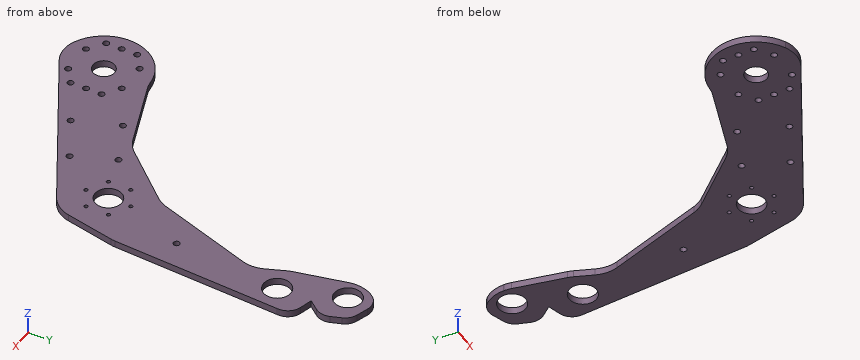
```python
from build123d import *

# Parameters (mm, degrees)
SKETCH1_R           = 8.89
SKETCH1_R_2         = 10.9347
SKETCH1_R_3         = 11.1125
SKETCH1_R_4         = 1.524
SKETCH1_R_5         = 2.5
SKETCH1_R_6         = 2.54
BOSS_EXTRUDE1_DEPTH = 5.55625
FILLET1_R           = 25.4
FILLET3_R           = 12.7
FILLET4_R           = 12.7


with BuildPart() as part:
    # Sketch1 → Boss-Extrude1 (new body)
    with BuildSketch(Plane.XY):
        with BuildLine():
            Line((199.79602437, 71.078107547), (188.964925061, 57.285610842))
            Line((188.964925061, 57.285610842), (206.456809173, 52.506453094))
            Line((206.456809173, 52.506453094), (208.830818929, 45.887219752))
            Line((208.830818929, 45.887219752), (200.684125291, -98.616772294))
            Line((200.684125291, -98.616772294), (189.611167808, -151.385643895))
            Line((189.611167808, -151.385643895), (38.107034572, -236.120024372))
            ThreePointArc((38.107034572, -236.120024372), (1.581834572, -199.594824372), (38.107034572, -163.069624372))
            Line((38.107034572, -163.069624372), (103.261818833, -139.701647224))
            Line((103.261818833, -139.701647224), (147.550432491, -89.7457244))
            Line((147.550432491, -89.7457244), (171.836242771, -16.814689905))
            Line((171.836242771, -16.814689905), (178.189444477, 2.26417003))
            Line((178.189444477, 2.26417003), (167.830043749, 27.447208055))
            Line((167.830043749, 27.447208055), (157.470643022, 73.010133983))
            Line((157.470643022, 73.010133983), (157.470643022, 93.390021886))
            Line((157.470643022, 93.390021886), (170.600142232, 98.791028052))
            Line((170.600142232, 98.791028052), (192.468434241, 91.508954042))
            Line((192.468434241, 91.508954042), (199.79602437, 71.078107547))
        make_face()
        with Locations((38.107034572, -199.594824372)):
            Circle(SKETCH1_R, mode=Mode.SUBTRACT)
        with Locations((161.671727665, -124.770570211)):
            Circle(SKETCH1_R_2, mode=Mode.SUBTRACT)
        with Locations((188.964925061, 29.396113336)):
            Circle(SKETCH1_R_3, mode=Mode.SUBTRACT)
        with Locations((173.035965272, 78.237579188)):
            Circle(SKETCH1_R_3, mode=Mode.SUBTRACT)
        with Locations((161.671727665, -106.355570211)):
            Circle(SKETCH1_R_4, mode=Mode.SUBTRACT)
        with Locations((12.721199582, -186.891028869)):
            Circle(SKETCH1_R_5, mode=Mode.SUBTRACT)
        with Locations((177.619585475, -115.563070211)):
            Circle(SKETCH1_R_4, mode=Mode.SUBTRACT)
        with Locations((177.619585475, -133.978070211)):
            Circle(SKETCH1_R_4, mode=Mode.SUBTRACT)
        with Locations((161.671727665, -143.185570211)):
            Circle(SKETCH1_R_4, mode=Mode.SUBTRACT)
        with Locations((145.723869854, -133.978070211)):
            Circle(SKETCH1_R_4, mode=Mode.SUBTRACT)
        with Locations((145.723869854, -115.563070211)):
            Circle(SKETCH1_R_4, mode=Mode.SUBTRACT)
        with Locations((12.721199582, -199.591028869)):
            Circle(SKETCH1_R_5, mode=Mode.SUBTRACT)
        with Locations((12.721199582, -212.291028869)):
            Circle(SKETCH1_R_5, mode=Mode.SUBTRACT)
        with Locations((25.421199582, -221.588074125)):
            Circle(SKETCH1_R_5, mode=Mode.SUBTRACT)
        with Locations((25.421199582, -177.593983613)):
            Circle(SKETCH1_R_5, mode=Mode.SUBTRACT)
        with Locations((50.821199582, -177.593983613)):
            Circle(SKETCH1_R_5, mode=Mode.SUBTRACT)
        with Locations((63.521199582, -186.891028869)):
            Circle(SKETCH1_R_5, mode=Mode.SUBTRACT)
        with Locations((63.521199582, -199.591028869)):
            Circle(SKETCH1_R_5, mode=Mode.SUBTRACT)
        with Locations((63.521199582, -212.291028869)):
            Circle(SKETCH1_R_5, mode=Mode.SUBTRACT)
        with Locations((50.821199582, -221.588074125)):
            Circle(SKETCH1_R_5, mode=Mode.SUBTRACT)
        with Locations((181.29246285, -57.510690342)):
            Circle(SKETCH1_R_6, mode=Mode.SUBTRACT)
        with Locations((99.96903305, -191.23088449)):
            Circle(SKETCH1_R_6, mode=Mode.SUBTRACT)
        with Locations((134.782371312, -172.083548446)):
            Circle(SKETCH1_R_6, mode=Mode.SUBTRACT)
        with Locations((121.031102699, -139.896498857)):
            Circle(SKETCH1_R_6, mode=Mode.SUBTRACT)
        with Locations((86.391831128, -156.243479537)):
            Circle(SKETCH1_R_6, mode=Mode.SUBTRACT)
    extrude(amount=BOSS_EXTRUDE1_DEPTH)

    # Fillet1
    # the kernel refuses this fillet: 25.4 mm, written as the material it adds along each edge
    with BuildSketch(Plane(origin=(178.189444477, 2.26417003, 0), x_dir=(-0.38043310119112633, 0.9248084426074961, 0), z_dir=(0, 0, 1))) as fillet1_piece_1:
        with BuildLine():
            CenterArc((FILLET1_R * 0.371679258358, FILLET1_R), FILLET1_R, 229.221887669, 40.778112331)
            Line((-FILLET1_R * 0.281452116845, FILLET1_R * 0.242755385146), (0, 0))
            Line((0, 0), (FILLET1_R * 0.371679258358, 0))
        make_face()
    extrude(amount=5.55625)
    with BuildSketch(Plane(origin=(147.550432491, -89.7457244, 0), x_dir=(0.3159404927300864, 0.9487790074898739, 0), z_dir=(0, 0, 1))) as fillet1_piece_2:
        with BuildLine():
            CenterArc((FILLET1_R * 0.204735054156, FILLET1_R), FILLET1_R, 246.858885181, 23.141114819)
            Line((-FILLET1_R * 0.188262015137, FILLET1_R * 0.0804602762649), (0, 0))
            Line((0, 0), (FILLET1_R * 0.204735054156, 0))
        make_face()
    extrude(amount=5.55625)
    with BuildSketch(Plane(origin=(103.261818833, -139.701647224, 0), x_dir=(0.6633872027522849, 0.7482762987189282, 0), z_dir=(0, 0, 1))) as fillet1_piece_3:
        with BuildLine():
            CenterArc((FILLET1_R * 0.255926298649, FILLET1_R), FILLET1_R, 241.289253159, 28.710746841)
            Line((-FILLET1_R * 0.224461714683, FILLET1_R * 0.122943926167), (0, 0))
            Line((0, 0), (FILLET1_R * 0.255926298649, 0))
        make_face()
    extrude(amount=5.55625)
    with BuildSketch(Plane(origin=(38.107034572, -163.069624372, 0), x_dir=(-0.999191470019892, -0.040204554959449905, 0), z_dir=(0, 0, 1))) as fillet1_piece_4:
        with BuildLine():
            CenterArc((3.958154518, -25.379463339), FILLET1_R, 92.304172347, 15.122193833)
            Line((-3.648634427, -1.145256895), (0, 0))
            ThreePointArc((0, 0), (1.468479411, -0.029531719), (2.936958822, 0))
        make_face()
    extrude(amount=5.55625)
    # the kernel refuses this fillet: 25.4 mm, written as the material it takes off along each edge
    with BuildSketch(Plane(origin=(157.470643022, 93.390021886, -42.096203676), x_dir=(0, -1, 0), z_dir=(0, 0, 1))) as fillet1_2_piece_1:
        with BuildLine():
            CenterArc((16.83848147, 25.4), FILLET1_R, 208.887448124, 61.112551876)
            Line((-5.401006167, 13.12949921), (0, 0))
            Line((0, 0), (16.83848147, 0))
        make_face()
    extrude(amount=89.748657352, mode=Mode.SUBTRACT)
    with BuildSketch(Plane(origin=(157.470643022, 73.010133983, -7.12787144), x_dir=(0.2217063764510564, -0.9751134716744213, 0), z_dir=(0, 0, 1))) as fillet1_2_piece_2:
        with BuildLine():
            CenterArc((FILLET1_R * 0.11224994393, FILLET1_R), FILLET1_R, 257.190723516, 12.809276484)
            Line((-FILLET1_R * 0.109456432521, FILLET1_R * 0.0248865283256), (0, 0))
            Line((0, 0), (FILLET1_R * 0.11224994393, 0))
        make_face()
    extrude(amount=19.811992879, mode=Mode.SUBTRACT)
    with BuildSketch(Plane(origin=(167.830043749, 27.447208055, -5.305032246), x_dir=(0.38043310119112356, -0.9248084426074973, 0), z_dir=(0, 0, 1))) as fillet1_2_piece_3:
        with BuildLine():
            CenterArc((FILLET1_R * 0.0835438149047, FILLET1_R), FILLET1_R, 260.448763965, 9.551236035)
            Line((-FILLET1_R * 0.0823856984158, FILLET1_R * 0.0138623845481), (0, 0))
            Line((0, 0), (FILLET1_R * 0.0835438149047, 0))
        make_face()
    extrude(amount=16.166314493, mode=Mode.SUBTRACT)
    with BuildSketch(Plane(origin=(38.107034572, -236.120024372, -39.792317969), x_dir=(-0.975973408380196, 0.21788966504803134, 0), z_dir=(0, 0, 1))) as fillet1_2_piece_4:
        with BuildLine():
            CenterArc((10.382529695, -24.789724573), FILLET1_R, 77.414886959, 54.38796922)
            Line((-6.548338937, -5.855478157), (0, 0))
            ThreePointArc((0, 0), (7.958463594, 0.877576064), (15.916927188, 0))
        make_face()
    extrude(amount=85.140885938, mode=Mode.SUBTRACT)
    with BuildSketch(Plane(origin=(189.611167808, -151.385643895, -28.892669195), x_dir=(-0.8727709569033328, -0.4881299589105759, 0), z_dir=(0, 0, 1))) as fillet1_2_piece_5:
        with BuildLine():
            CenterArc((FILLET1_R * 0.455002664481, -FILLET1_R), FILLET1_R, 90, 48.931323179)
            Line((-FILLET1_R * 0.298919997384, -FILLET1_R * 0.343036819962), (0, 0))
            Line((0, 0), (FILLET1_R * 0.455002664481, 0))
        make_face()
    extrude(amount=63.341588389, mode=Mode.SUBTRACT)
    with BuildSketch(Plane(origin=(200.684125291, -98.616772294, -4.788068762), x_dir=(0.056287565067425785, 0.9984145982600516, 0), z_dir=(0, 0, 1))) as fillet1_2_piece_6:
        with BuildLine():
            CenterArc((FILLET1_R * 0.0754026576756, FILLET1_R), FILLET1_R, 261.375811644, 8.624188356)
            Line((-FILLET1_R * 0.0745500922014, FILLET1_R * 0.0113068358665), (0, 0))
            Line((0, 0), (FILLET1_R * 0.0754026576756, 0))
        make_face()
    extrude(amount=15.132387525, mode=Mode.SUBTRACT)
    with BuildSketch(Plane(origin=(208.830818929, 45.887219752, -12.894572268), x_dir=(-0.3375970122965893, 0.9412907400417878, 0), z_dir=(0, 0, 1))) as fillet1_2_piece_7:
        with BuildLine():
            CenterArc((FILLET1_R * 0.203064130199, FILLET1_R), FILLET1_R, 247.042716146, 22.957283854)
            Line((-FILLET1_R * 0.186980618985, FILLET1_R * 0.0792040977315), (0, 0))
            Line((0, 0), (FILLET1_R * 0.203064130199, 0))
        make_face()
    extrude(amount=31.345394535, mode=Mode.SUBTRACT)

    # Fillet3
    fillet3_edges = [part.edges().sort_by_distance(p)[0] for p in [
        (170.600142232, 98.791028052, 2.778125),
        (192.468434241, 91.508954042, 2.778125),
    ]]
    fillet(fillet3_edges, radius=FILLET3_R)

    # Fillet4
    fillet4_edges = [part.edges().sort_by_distance(p)[0] for p in [
        (206.456809173, 52.506453094, 2.778125),
        (199.79602437, 71.078107547, 2.778125),
    ]]
    fillet(fillet4_edges, radius=FILLET4_R)


solid = part.part
```
Build history of the part. All positions in model axes, mm. Round coordinates to 2 decimals unless told otherwise and drop trailing zeros. Write each loop counter-clockwise with the first axis right and the second up, starting at its lowest first coordinate (ties: lowest second). Pieces come first, ordered by that corner, then holes. Notation, with made-up numbers: (42, 3.5) -> (53, 3.5) arc R10 cw to (53, 20.5) -> close; hole circle Ø7 at (72, -34.5). An arc over 180 degrees is marked (long way). Put each result on its own line as item: value.
Item 1: Slice it at C-C, the plane y = -43.5. Give the cut face in (x, z), plus the area to 3 significant figures.
Here are the results:
outline: (162.95, 0) -> (203.79, 0) -> (203.79, 5.56) -> (162.95, 5.56) -> close
area: 227 mm^2
Item 2: Flat gauge pins, fed straight in: P1, Ø3, axis at x = 134.78, y = -172.08, coming from the +Z side; P2, Ø2, axis at y = 8, z = 4, coming from the +X side; P3, Ø3, axis at x = 33, z = 4.5, coming from the +Y side; P4, Ø1.5, axis at y = -62.5, z = 4.5, coming from the +X side. Where does each tip first touch, or does it go through?
Here are the results:
P1: passes through
P2: stops at x = 206.75
P3: stops at y = -163.25
P4: stops at x = 202.76
Item 3: Slice it at A-A, the plane z = 2.6. Count the separate pieces of the cut face and the enclosed holes in it, plus the area to 3 significant figures.
Here are the results:
separate pieces: 1
enclosed holes: 25
area: 18,600 mm^2
Item 4: Wall check: probe 1 along Y at (x, z) = (27, 3.75); probe 2 along Y at (x, z) = (65.5, 0.6); probe 3 along Y at (x, z) = (13, 3.1). Give the ranges that are in metal, low to high. Write a range as from..to.
Here are the results:
probe 1: y = -234.25..-223.53, -219.65..-179.53, -175.66..-164.8
probe 2: y = -220.8..-213.82, -210.76..-201.12, -198.06..-188.42, -185.36..-153.25
probe 3: y = -226.12..-214.78, -209.81..-202.08, -197.11..-189.38, -184.41..-173.07
Item 5: Slice it at B-B, the plane x = 93. Give the cut face in (y, z).
Here are the results:
outline: (-205.42, 0) -> (-143.38, 0) -> (-143.38, 5.56) -> (-205.42, 5.56) -> close
